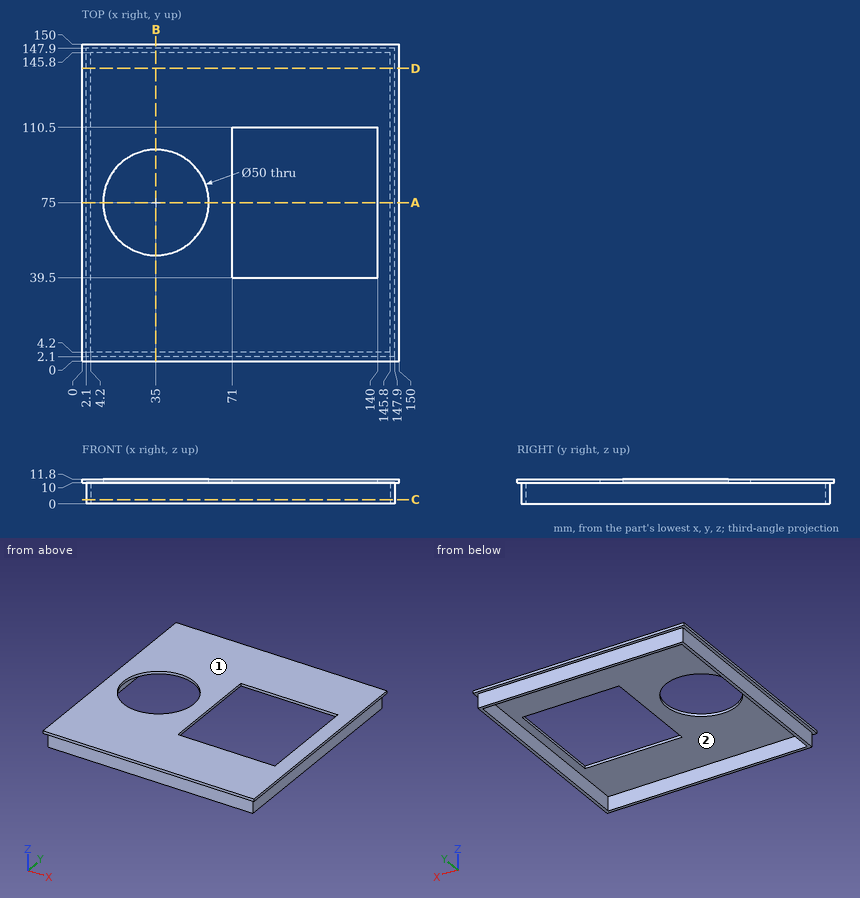
Check sheet for the drawn part. Datum: minimum x, y, z corner. Units: mm. Give positions to 0.01 mm unless a question says otherwise; leave off trailing zeros. Write each loop counter-clockwise with the first axis right and the second up, starting at its lowest first coordinate (ties: lowest second). Pieces come first, ordered by that corner, then holes. Notation, with made-up numbers: (76.5, 6.5) -> (99.5, 6.5) arc R14 ccw to (99.5, 33.5) -> close; hole circle Ø8 at (9.25, 15.25). An arc over 180 degrees is marked (long way). Use one line per item in the form item = value. Start each with the question number.
1. Mould release check, pull along Y, two halves, no side actions. Record for the marked faces 1 and 2: pulls with the +Y half, pulls with the -Y half, needs draft (parallel to the pull), parting line crosses it, or undercut.
2. Section check D-D (y = 138.5). Record the cut outline in (x, z).
3. Go/stop test with flat-tipped pins: P1, Ø3, axis at x = 103, z = 7, coming from the -Y side; P2, Ø5, axis at y = 96, z = 5.5, coming from the +X side. Record where each tip stops, or that it passes through.
4. Thickness scan on line 1 along Y through (x, z) = (35, 10.6); line 2 along Y through (x, z) = (97.5, 4.25). Record the ranges inside material, lowest first. Write a range as from..to.
5. Section check A-A (y = 75). Record the cut outline in (x, z).
6. Section check C-C (z = 2). Record the cut outline in (x, y).
7. Section check B-B (x = 35). Record the cut outline in (y, z).
Conclusion:
q1.face_1 = needs draft
q1.face_2 = undercut
q2.outline = (0, 10) -> (2.1, 10) -> (2.1, 0) -> (4.2, 0) -> (4.2, 10) -> (145.8, 10) -> (145.8, 0) -> (147.9, 0) -> (147.9, 10) -> (150, 10) -> (150, 11.8) -> (0, 11.8) -> close
q3.P1 = 2.1
q3.P2 = 147.9
q4.line_1 = 0..50, 100..150
q4.line_2 = 2.1..4.2, 145.8..147.9
q5.outline = (0, 10) -> (2.1, 10) -> (2.1, 0) -> (4.2, 0) -> (4.2, 10) -> (10, 10) -> (10, 11.8) -> (0, 11.8) -> close; (60, 10) -> (71, 10) -> (71, 11.8) -> (60, 11.8) -> close; (140, 10) -> (145.8, 10) -> (145.8, 0) -> (147.9, 0) -> (147.9, 10) -> (150, 10) -> (150, 11.8) -> (140, 11.8) -> close
q6.outline = (2.1, 2.1) -> (147.9, 2.1) -> (147.9, 147.9) -> (2.1, 147.9) -> close; hole (4.2, 4.2) -> (145.8, 4.2) -> (145.8, 145.8) -> (4.2, 145.8) -> close
q7.outline = (0, 10) -> (2.1, 10) -> (2.1, 0) -> (4.2, 0) -> (4.2, 10) -> (50, 10) -> (50, 11.8) -> (0, 11.8) -> close; (100, 10) -> (145.8, 10) -> (145.8, 0) -> (147.9, 0) -> (147.9, 10) -> (150, 10) -> (150, 11.8) -> (100, 11.8) -> close
